Design review of the part built by this model. Coordinates are the model's own, in mm. Face numbers are marked on the shaded views. Give positions to 0.01 mm unless a question says otherwise; leave off trailing zeros. Write each loop counter-clockwise with the first axis right and the second up, starting at its lowest first coordinate (ties: lowest second). Pieces come first, ordered by that corner, then holes. Notation, with made-up numbers: M 31.5,24.25 L 52.5,24.25 A12 cw 52.5,47.25 Z; hole C -14.75,50.25 d5. An arc over 180 degrees is marked long. Use a Markdown table: item, result. Add a question column.
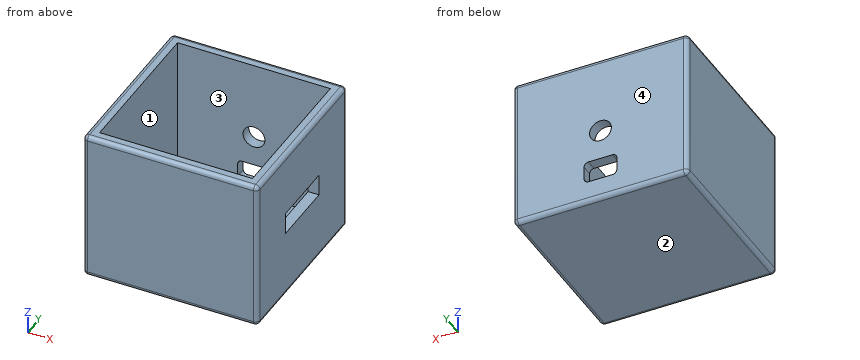
```python
from build123d import *

# Parameters (mm, degrees)
SKETCH_1_W          = 80
SKETCH_1_H          = 80
EXTRUDE_1_DEPTH     = 70
SKETCH_2_W          = 70
SKETCH_2_H          = 70
CUT_EXTRUDE_1_DEPTH = 65
FILLET_1_R          = 2
FILLET_2_R          = 2
FILLET_3_R          = 2
CUT_EXTRUDE_3_DEPTH = 10
SKETCH_4_W          = 10
SKETCH_4_H          = 30
CUT_EXTRUDE_4_DEPTH = 10
SKETCH_5_R          = 5
CUT_EXTRUDE_5_DEPTH = 10
FILLET_4_R          = 2


with BuildPart() as part:
    # Эскиз1 → Бобышка-Вытянуть1 (new body)
    with BuildSketch(Plane.XY):
        Rectangle(SKETCH_1_W, SKETCH_1_H)
    extrude(amount=EXTRUDE_1_DEPTH)

    # Эскиз2 → Вырез-Вытянуть1 (cut)
    with BuildSketch(Plane.XY.offset(70)):
        Rectangle(SKETCH_2_W, SKETCH_2_H)
    extrude(amount=-CUT_EXTRUDE_1_DEPTH, mode=Mode.SUBTRACT)

    # Скругление1
    fillet_1_edges = [part.edges().sort_by_distance(p)[0] for p in [
        (-40, 40, 35),
        (-40, -40, 35),
    ]]
    fillet(fillet_1_edges, radius=FILLET_1_R)

    # Скругление2
    fillet_2_edges = [part.edges().sort_by_distance(p)[0] for p in [
        (1, -40, 0),
        (-40, 0, 0),
        (-39.414213562, 39.414213562, 0),
        (-39.414213562, -39.414213562, 0),
        (1, 40, 0),
        (40, 0, 0),
        (40, 40, 35),
    ]]
    fillet(fillet_2_edges, radius=FILLET_2_R)

    # Скругление3
    # the kernel refuses this fillet: 2 mm, written as the material it takes off along each edge
    with BuildSketch(Plane(origin=(38, -38, 2), x_dir=(1, 0, 0), z_dir=(0, -1, 0))) as fillet_3_piece_1_section:
        Polygon((0, 0), (FILLET_3_R, 0), (FILLET_3_R, -FILLET_3_R), (0, -FILLET_3_R), align=None)
    fillet_3_piece_1 = extrude(amount=FILLET_3_R, mode=Mode.PRIVATE)
    fillet_3_piece_1 = fillet_3_piece_1 - Plane(origin=(38, -38, 2), x_dir=(-0.7071067811865475, 0, 0.7071067811865475), z_dir=(0, -1, 0)) * Sphere(FILLET_3_R, mode=Mode.PRIVATE)
    add(fillet_3_piece_1, mode=Mode.SUBTRACT)
    with BuildSketch(Plane(origin=(40, -40, 2), x_dir=(-1, 0, 0), z_dir=(0, 0, 1))) as fillet_3_piece_2:
        with BuildLine():
            CenterArc((FILLET_3_R, -FILLET_3_R), FILLET_3_R, 90, 90)
            Line((0, -FILLET_3_R), (0, 0))
            Line((0, 0), (FILLET_3_R, 0))
        make_face()
    extrude(amount=73, mode=Mode.SUBTRACT)

    # Эскиз3 → Вырез-Вытянуть3 (cut)
    with BuildSketch(Plane(origin=(0, 40, 0), x_dir=(1, 0, 0), z_dir=(0, 1, 0))):
        with BuildLine():
            Line((5.5, -20), (-5.5, -20))
            ThreePointArc((-5.5, -20), (-6.914213562, -19.414213562), (-7.5, -18))
            Line((-7.5, -18), (-7.5, -12))
            ThreePointArc((-7.5, -12), (-6.914213562, -10.585786438), (-5.5, -10))
            Line((-5.5, -10), (5.5, -10))
            ThreePointArc((5.5, -10), (6.914213562, -10.585786438), (7.5, -12))
            Line((7.5, -12), (7.5, -18))
            ThreePointArc((7.5, -18), (6.914213562, -19.414213562), (5.5, -20))
        make_face()
    extrude(amount=-CUT_EXTRUDE_3_DEPTH, mode=Mode.SUBTRACT)

    # Эскиз4 → Вырез-Вытянуть4 (cut)
    with BuildSketch(Plane(origin=(40, 0, 0), x_dir=(0, 0, -1), z_dir=(1, 0, 0))):
        with Locations((-36, 0)):
            Rectangle(SKETCH_4_W, SKETCH_4_H)
    extrude(amount=-CUT_EXTRUDE_4_DEPTH, mode=Mode.SUBTRACT)

    # Эскиз5 → Вырез-Вытянуть5 (cut)
    with BuildSketch(Plane(origin=(0, 40, 0), x_dir=(1, 0, 0), z_dir=(0, 1, 0))):
        with Locations(Location((0, -34, 0), (0, 0, 270))):
            Circle(SKETCH_5_R)
    extrude(amount=-CUT_EXTRUDE_5_DEPTH, mode=Mode.SUBTRACT)

    # Скругление4
    fillet_4_edges = [part.edges().sort_by_distance(p)[0] for p in [
        (0, -40, 70),
        (-40, 0, 70),
        (-39.414213562, 39.414213562, 70),
        (-39.414213562, -39.414213562, 70),
        (0, 40, 70),
        (39.414213562, 39.414213562, 70),
        (40, 0, 70),
        (39.414213562, -39.414213562, 70),
    ]]
    fillet(fillet_4_edges, radius=FILLET_4_R)


solid = part.part
```
(1) Add section A-A on z = 34. Give the boundary of the cut face in (x, y), then the cut area to 3 significant figures.
(2) Add section C-C on y = -23. Give the boundary of the cut face in (x, z), then the cut area to 3 significant figures.
(3) For pin 1 (1 mm diameter, centred on x = -10.5, y = 6.5, fed in from +Z), flat-tipped, find the tip position at first contact; note if it passes through.
(4) Wall thickness on L1, parallel to X at y = -10.5, z = 12; L2, parallel to X at y = 38.1, z = 34: over which ranges is each line inside the solid? List them lowest first.
(5) The part is to be moulded in two halves that separate along Y. For the marked faces 1, 2, 3 and 4, say which applies: released by +Y, released by -Y, zero draft, split by the parting line, or undercut.
(6) Add section B-B on x = 0. Give the boundary of the cut face in (y, z), then the cut area to 3 significant figures.
From the geometry:
| question | item | result |
|---|---|---|
| 1 | outline | M -40,-38 A2 ccw -38,-40 L 38,-40 A2 ccw 40,-38 L 40,-15 L 35,-15 L 35,-35 L -35,-35 L -35,35 L -5,35 L -5,40 L -38,40 A2 ccw -40,38 Z; M 5,35 L 35,35 L 35,15 L 40,15 L 40,38 A2 ccw 38,40 L 5,40 Z |
| 1 | area | 1,300 mm^2 |
| 2 | outline | M -40,2 A2 ccw -38,0 L 38,0 A2 ccw 40,2 L 40,68 A2 ccw 38,70 L 35,70 L 35,5 L -35,5 L -35,70 L -38,70 A2 ccw -40,68 Z |
| 2 | area | 1,050 mm^2 |
| 3 | pin 1 | stops at z = 5 |
| 4 | L1 | x = -40 to -35, 35 to 40 |
| 4 | L2 | x = -40 to -5, 5 to 40 |
| 5 | face 1 | undercut |
| 5 | face 2 | zero draft |
| 5 | face 3 | undercut |
| 5 | face 4 | released by +Y |
| 6 | outline | M -40,2 A2 ccw -38,0 L 38,0 A2 ccw 40,2 L 40,10 L 35,10 L 35,5 L -35,5 L -35,70 L -38,70 A2 ccw -40,68 Z; M 35,20 L 40,20 L 40,29 L 35,29 Z; M 35,39 L 40,39 L 40,68 A2 ccw 38,70 L 35,70 Z |
| 6 | area | 947 mm^2 |
